Input: part model. Units: mm. Frame: model coordinates. A direction names the side the tool comes from. Round coordinates to 2 decimals unless told otherwise and drop trailing zeros. Write each loop counter-clockwise with the first axis right and the second up, starting at its lowest first coordinate (ties: lowest second). Pieces come first, ordered by that corner, then holes. Notation, with made-up numbers: M 39,88.25 L 43,88.25 A18 ccw 43,96.25 Z; hole C -20.75,35.25 d7. An arc over 180 degrees is marked long. Use one line per item in the form item = value. Start each with the question number.
```python
from build123d import *

# Parameters (mm, degrees)
BOSS_EXTRU_1_DEPTH                                   = 10
CHAMBRAGE_POUR_T_TE_CYLINDRIQUE_FENDUE_M_D           = 4
CHAMBRAGE_POUR_T_TE_CYLINDRIQUE_FENDUE_M_CBORE_D     = 5.5
CHAMBRAGE_POUR_T_TE_CYLINDRIQUE_FENDUE_M_CBORE_DEPTH = 4
ESQUISSE6_R                                          = 2
ENL_V_MAT_EXTRU_1_DEPTH                              = 90.844829046


with BuildPart() as part:
    # Esquisse1 → Boss.-Extru.1 (new body)
    with BuildSketch(Plane(origin=(0, 0, 0), x_dir=(1, 0, 0), z_dir=(0, 1, 0))):
        Polygon((63.135145942, -29.291431628), (63.135145942, 29.291431628), (29.291431628, 63.135145942), (-29.291431628, 63.135145942), (-63.135145942, 29.291431628), (-63.135145942, -29.291431628), (-29.291431628, -63.135145942), (29.291431628, -63.135145942), align=None)
    extrude(amount=BOSS_EXTRU_1_DEPTH)

    # Chambrage pour tête cylindrique fendue M31 (through all)
    with Locations(Plane(origin=(-28.889172646, 10, -52.930803206), x_dir=(0, 0, 1), z_dir=(0, 1, 0))):
        with Locations((0, 0), (24.04163056, -24.04163056), (81.819975852, -24.04163056), (105.861606412, 0), (105.861606412, 57.778345292), (81.819975852, 81.819975852), (24.04163056, 81.819975852), (0, 57.778345292)):
            CounterBoreHole(CHAMBRAGE_POUR_T_TE_CYLINDRIQUE_FENDUE_M_D / 2, CHAMBRAGE_POUR_T_TE_CYLINDRIQUE_FENDUE_M_CBORE_D / 2, CHAMBRAGE_POUR_T_TE_CYLINDRIQUE_FENDUE_M_CBORE_DEPTH)

    # Esquisse6 → Enlèv. mat.-Extru.1 (cut, through all)
    with BuildSketch(Plane.XZ):
        with Locations(Location((-44.194173824, 9.545941546, 0), (0, 0, 270))):
            Circle(ESQUISSE6_R)
        with Locations(Location((-9.545941546, 44.194173824, 0), (0, 0, 270))):
            Circle(ESQUISSE6_R)
        with Locations(Location((-3.181980515, -31.466251763, 0), (0, 0, 270))):
            Circle(ESQUISSE6_R)
        with Locations(Location((31.466251763, 3.181980515, 0), (0, 0, 270))):
            Circle(ESQUISSE6_R)
        with Locations(Location((28.677040611, 38.293692836, 0), (0, 0, 270))):
            Circle(ESQUISSE6_R)
        with Locations(Location((38.293692836, 28.677040611, 0), (0, 0, 270))):
            Circle(ESQUISSE6_R)
    extrude(amount=-ENL_V_MAT_EXTRU_1_DEPTH, mode=Mode.SUBTRACT)


solid = part.part
```
Item 1: Reachability of faces 5 (the face through (-4.4, 4.93, -29.88)), 6 (the face through (-31, 6, 52)) from +Z, -Z, +X, -X, +Y, -Y: full face, straight path, thin tool, end or side. Return the list, or none.
Item 2: Cut plane B-B (z = -35). Output: boundary loops of the cut face in (x, y), plus the area to 3 significant figures.
Item 3: Cut plane A-A (y = 3.75). Give the number of separate pieces and of enclosed holes in the cut face, plus the area to 3 significant figures.
Item 4: First-contact query: pin 1 (3.5 mm diameter, centred on x = 52.93, z = 28.89, fed in from +Y); pin 2 (5 mm diameter, centred on x = -52.93, z = 28.89, fed in from +Y). Flat tips, straight axial feed; report the tip coordinate or a pass-through.
Item 5: Draft query along X for faces 1 (the face through (51.88, 8.03, 31.43)), 2 (the face through (0, 5, -63.135)), 3 (the face through (-45.976, 4.93, -46.45)), 4 (the face through (-50.612, 8.028, -27.411)). Return one class per face: +X half, -X half, draft (parallel to the pull), parting line (faces both ways), or undercut.
Item 6: Ray query, line 1 (Z direction, x = -54, y = 9); line 2 (Z direction, x = -52, y = 6.25); line 3 (X direction, y = 3.75, z = -30). Return the intervals inside material, ascending. Write a range as from..to.
Item 7: Cut plane C-C (z = 34.5). Output: boundary loops of the cut face in (x, y).
Final values:
q1.face_5 = +Y, -Y
q1.face_6 = +Y
q2.outline = M -57.43,0 L 57.43,0 L 57.43,10 L -57.43,10 Z
q2.area = 1,150 mm^2
q3.separate_pieces = 1
q3.enclosed_holes = 14
q3.area = 13,500 mm^2
q4.pin_1 = through
q4.pin_2 = 6
q5.face_1 = undercut
q5.face_2 = draft
q5.face_3 = -X half
q5.face_4 = undercut
q6.line_1 = -38.43..-31.42, -26.36..26.36, 31.42..38.43
q6.line_2 = -40.43..-31.48, -26.3..26.3, 31.48..40.43
q6.line_3 = -62.43..-54.59, -51.27..-4.54, -1.82..51.27, 54.59..62.43
q7.outline = M -57.93,0 L 57.93,0 L 57.93,10 L -57.93,10 Z
